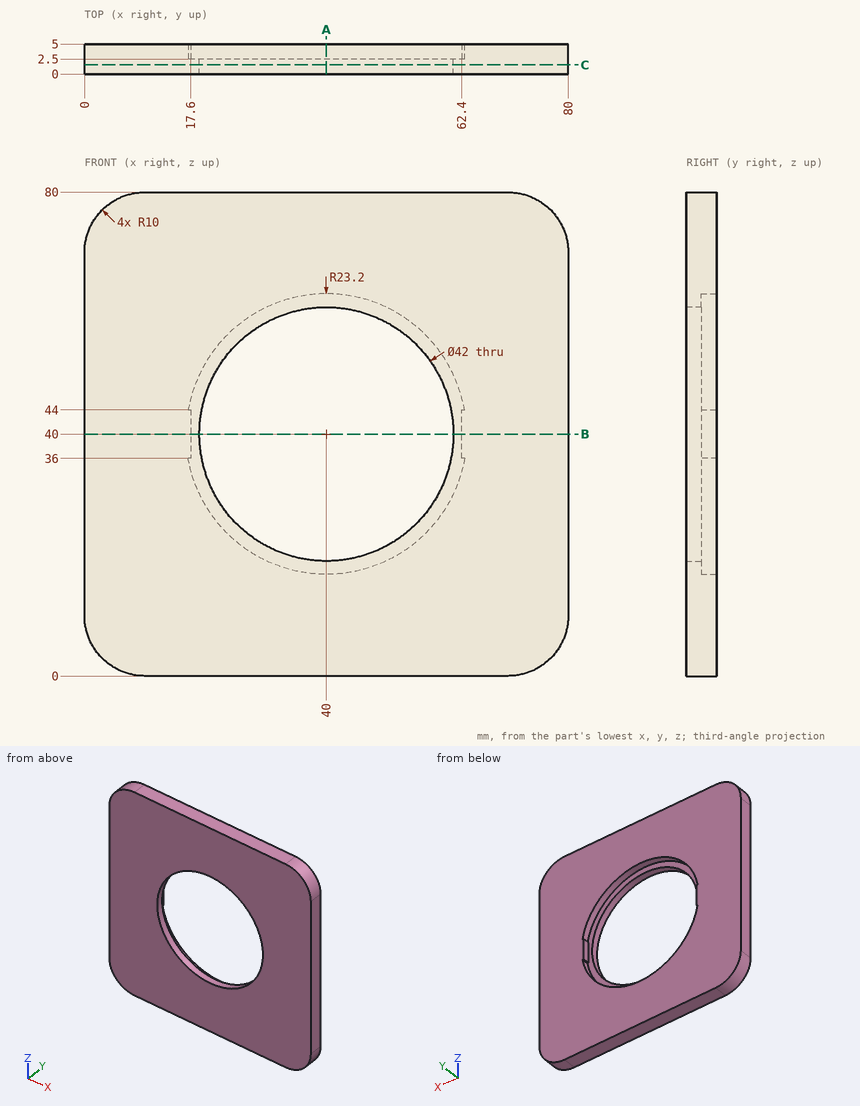
Answer from the drawing. Dimensions are ordinates in mm from the lowest x, y and z of the part. Coordinates: 2 decimals unless noted, no trailing zeros. Write each loop counter-clockwise with the first axis right and the second up, starting at its lowest first coordinate (ties: lowest second). Pieces come first, ordered by that corner, then holes. Notation, with made-up numbers: M -20.75,55 L -11.75,55 A18 cw -11.75,62 Z; hole C -23.75,89 d1. An arc over 180 degrees is marked long. Write item = value, one per line.
1. Straight lines are drawn through the part: line 1 (X direction, y = 1.85, z = 40); line 2 (X direction, y = 4.4, z = 39); line 3 (Z direction, x = 36, y = 2.2). For each, find the intervals that lie inside material, in ascending order. Write a range as from..to.
Solution:
line_1 = 0..19, 61..80
line_2 = 0..17.6, 62.4..80
line_3 = 0..19.38, 60.62..80
2. A flat-ended cylindrical pin translates along its axis: pin 1 (25 mm diameter, centred on x = 40, z = 40, fed in from +Y). Find the tip coordinate at first contact, or state that the pin passes through.
Solution:
pin_1 = through
3. The part is cut by section B-B (z = 40). Determine the outline of the cut face in (x, y), then the cut area to 3 significant figures.
Solution:
outline = M 0,0 L 19,0 L 19,2.5 L 17.6,2.5 L 17.6,5 L 0,5 Z; M 61,0 L 80,0 L 80,5 L 62.4,5 L 62.4,2.5 L 61,2.5 Z
area = 183 mm2
4. The part is cut by section C-C (y = 1.55). Determine the outline of the cut face in (x, z), then the cut area to 3 significant figures.
Solution:
outline = M 0,10 A10 ccw 10,0 L 70,0 A10 ccw 80,10 L 80,70 A10 ccw 70,80 L 10,80 A10 ccw 0,70 Z; hole C 40,40 d42
area = 4,930 mm2
5. The part is cut by section A-A (x = 40). Determine the outline of the cut face in (y, z).
Solution:
outline = M 0,0 L 5,0 L 5,16.8 L 2.5,16.8 L 2.5,19 L 0,19 Z; M 0,61 L 2.5,61 L 2.5,63.2 L 5,63.2 L 5,80 L 0,80 Z
